from build123d import *


with BuildPart() as part:
    # Sketch1 → Revolve1 (revolve)
    with BuildSketch(Plane.XY, mode=Mode.PRIVATE) as revolve1_sk:
        with BuildLine():
            Line((0, 5.5), (0, 14.67))
            Line((0, 14.67), (8, 14.67))
            Line((8, 14.67), (8, 13.17))
            Line((8, 13.17), (11, 13.17))
            Line((11, 13.17), (11, 20))
            Line((11, 20), (12, 20))
            ThreePointArc((12, 20), (16, 24), (20, 20))
            Line((20, 20), (20, 18))
            ThreePointArc((20, 18), (22.050252532, 13.050252532), (27, 11))
            Line((27, 11), (27, 5.5))
            Line((27, 5.5), (0, 5.5))
        make_face()
    revolve(revolve1_sk.sketch.rotate(Axis((0, 0, 0), (1, 0, 0)), 90), axis=Axis((0, 0, 0), (1, 0, 0)))

    # Ø3.5 (3.5) Diameter Hole2: read off the stored shape, not the designer's step
    # Ø3.5 (3.5) Diameter Hole2: loft between two sections, ruled curve by curve
    f_3_5_3_5_diameter_hole2_from = [
        Edge.make_three_point_arc((12.584394195, 4.719603739, -2.823958877), (13.87319466, 4.552306942, -0.717776277), (15.109619522, 2.611483824, -1.628522776)),
        Edge.make_three_point_arc((15.109619522, 2.611483824, -1.628522776), (13.820819057, 2.778780621, -3.734705376), (12.584394195, 4.719603739, -2.823958877)),
    ]
    f_3_5_3_5_diameter_hole2_to = [
        Edge.make_three_point_arc((21.045529414, 12.258443907, -7.402617534), (22.334329879, 12.09114711, -5.296434934), (23.570754741, 10.150323992, -6.207181432)),
        Edge.make_three_point_arc((23.570754741, 10.150323992, -6.207181432), (22.281954276, 10.317620789, -8.313364032), (21.045529414, 12.258443907, -7.402617534)),
    ]
    f_3_5_3_5_diameter_hole2 = Solid(Shell([*[Face.make_surface_from_curves(f_3_5_3_5_diameter_hole2_from[k], f_3_5_3_5_diameter_hole2_to[k]) for k in range(2)], Face(Wire(f_3_5_3_5_diameter_hole2_from)), Face(Wire(f_3_5_3_5_diameter_hole2_to))]))
    add(f_3_5_3_5_diameter_hole2, mode=Mode.SUBTRACT)


solid = part.part
Build history of the part. All positions in model axes, mm. A direction names the side the tool comes from. Coordinates: 2 decimals unless noted, no trailing zeros. Write each loop counter-clockwise with the first axis right and the second up, starting at its lowest first coordinate (ties: lowest second). Pieces come first, ordered by that corner, then holes.
(1) Cut at D-D on x = 9.25. List the corners of the cut face in (y, z).
(2) Mould opens along X. For faces 4 (the flat face through (8, -9, -10)), 5 (the cylindrical face through (4.06, 8.93, -11.64)), 6 (the flat face through (20, -3, -18)) say: pulls with the +X half, pulls with the -X half, needs draft (parallel to the pull), parting line crosses it, or undercut.
(3) Cut at A-A on y = 0. List the corners of the cut face in (x, z), and give its area (3 significant figures).
(4) 3-axis set-ups, long thin cutter, end or side, ignore diameter. For faces 1 (the flat face through (27, -3, -5)), 2 (the cylindrical face through (11.51, -0.88, -19.98)), 3 (the cylindrical face through (9.52, -3.96, 12.56)): which of +Z, -Z, +X, -X, +Y, -Y reach the whole face in a straight line?
(5) Pin check, flat tips, straight feed: pin 1 Ø1.5 at (x, z) = (23.5, -14.5) entering from -Y; pin 2 Ø17.5 at (y, z) = (0, 0) entering from -X; pin 3 Ø12 at (x, z) = (4, -0.5) entering from +Y; pin 4 Ø6 at (x, z) = (12.5, 6) entering from -Y. Stop position of each tip, or through.
(6) Drill centre lines: line 1 (Y direction, x = 6.5, z = 0); line 2 (Y direction, x = 6, z = 4); line 3 (Y direction, x = 25.5, z = -7). Where is each one in solid material? Low to high.
(7) Cut at C-C on x = 5.25. List the corners of the cut face in (y, z).
Working result:
1. outline: circle Ø26.34 at (0, 0); hole circle Ø11 at (0, 0)
2. face 4: undercut
2. face 5: needs draft
2. face 6: pulls with the +X half
3. outline: (0, -14.67) - (8, -14.67) - (8, -13.17) - (11, -13.17) - (11, -20) - (12, -20) arc R4 ccw to (20, -20) - (20, -18) arc R7 cw to (27, -11) - (27, -5.5) - (0, -5.5) - close; (0, 5.5) - (27, 5.5) - (27, 11) arc R7 cw to (20, 18) - (20, 20) arc R4 ccw to (12, 20) - (11, 20) - (11, 13.17) - (8, 13.17) - (8, 14.67) - (0, 14.67) - close
3. area: 602 mm2
4. face 1: +Z, -Z, +X, +Y, -Y
4. face 2: -X
4. face 3: none
5. pin 1: passes through
5. pin 2: stops at x = 0
5. pin 3: stops at y = 14.67
5. pin 4: stops at y = -23.48
6. line 1: y = -14.67 to -5.5, 5.5 to 14.67
6. line 2: y = -14.11 to -3.77, 3.77 to 14.11
6. line 3: y = -8.7 to 8.7
7. outline: circle Ø29.34 at (0, 0); hole circle Ø11 at (0, 0)
